from build123d import *

# Parameters (mm, degrees)
CYLINDER009_R             = 4.35
CYLINDER009_DEPTH         = 5.5
CYLINDER008_R             = 10.625
CYLINDER008_DEPTH         = 2.33
FUSION002_PLACEMENT_ANGLE = 90


with BuildPart() as servoplate002:
    # Cylinder009 → Cylinder009 (new body)
    with BuildSketch(Plane.XY):
        Circle(CYLINDER009_R)
    extrude(amount=CYLINDER009_DEPTH)


with BuildPart() as servoplate003:
    # Cylinder008 → Cylinder008 (new body)
    with BuildSketch(Plane.XY):
        Circle(CYLINDER008_R)
    extrude(amount=CYLINDER008_DEPTH)

    # Fusion002: union servoPlate002
    add(servoplate002.part)


with BuildPart() as servoplate003_1:
    # Fusion002 placement: moved
    add(servoplate003.part.moved(Location((18, 19, 20))).rotate(Axis((18, 19, 20), (1, 0, 0)), FUSION002_PLACEMENT_ANGLE))


solid = servoplate003_1.part
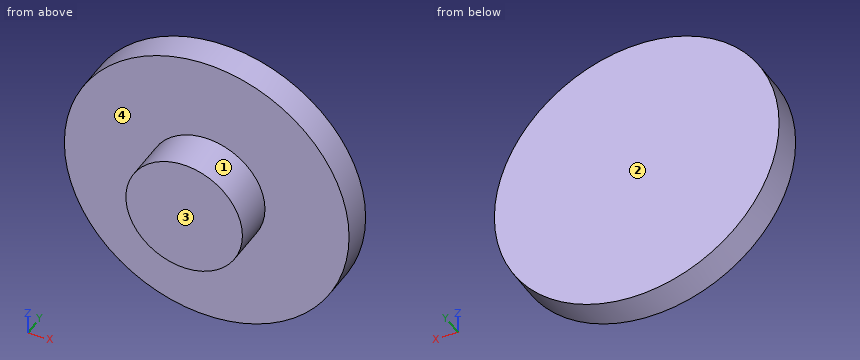
Verification items for the finished model (mm, model axes). Face numbers are marked on the shaded views. A direction names the side the tool comes from. Give positions to 0.01 mm unless a question says otherwise; leave off trailing zeros. Order: outer loops, then holes, each group sorted by start corner. A loop starts at its lowest first (then second) coordinate and runs counter-clockwise, first axis right, second up. Notation, with made-up numbers: M -20,50 L -2,50 A18 cw -2,61 Z; hole C 46.5,22 d10. An arc over 180 degrees is marked long. Use one line per item in the form item = value. Start each with the question number.
Q1. Scan lines: line 1 along Y through (x, z) = (14.25, 17.5); line 2 along X through (y, z) = (17.45, 15.25); line 3 along Z through (x, y) = (21, 16.35). Record each from-to range of solid material in increasing order. Write a range as [from, to].
Q2. Mould release check, pull along X, two halves, no side actions. Record for the marked faces 1 and 2: +X half, -X half, draft (parallel to the pull), parting line (faces both ways), or undercut.
Q3. Section check B-B (x = 18). Enter the section's corners in (y, z) (3 decimals).
Q4. Access from +Z, -Z, +X, -X, +Y, -Y to the whole of each face (thin tool, end or side, straight path). Record for the marked faces 3 and 4.
Q5. Section check D-D (y = 17). Enter the section's corners in (x, z) (3 decimals).
Q6. Section check A-A (z = 20). Enter the section's corners in (x, y) (3 decimals).
Q7. Section check C-C (y = 15.6). Enter the section's corners in (x, z).
Q8. Go/stop test with flat-tipped pins: pin 1 Ø1 at (x, z) = (11, 27) entering from -Y; pin 2 Ø10 at (x, z) = (21, 15.5) entering from -Y; pin 3 Ø2 at (y, z) = (15, 13) entering from -X. Record where each tip stops, or that it passes through.
Evaluation:
q1.line_1 = [16.67, 19]
q1.line_2 = [8.5, 27.5]
q1.line_3 = [16.85, 23.15]
q2.face_1 = parting line
q2.face_2 = draft
q3.outline = M 13.5,15.65 L 16.67,15.65 L 16.67,9.375 L 19,9.375 L 19,30.625 L 16.67,30.625 L 16.67,24.35 L 13.5,24.35 Z
q4.face_3 = +Z, -Z, +X, -X, -Y
q4.face_4 = -Y
q5.outline = C 18,20 d21.25
q6.outline = M 7.375,16.67 L 13.65,16.67 L 13.65,13.5 L 22.35,13.5 L 22.35,16.67 L 28.625,16.67 L 28.625,19 L 7.375,19 Z
q7.outline = C 18,20 d8.7
q8.pin_1 = 16.67
q8.pin_2 = 13.5
q8.pin_3 = through
